Model file for the job. Use its own axes, mm. Face numbers are marked on the shaded views. A direction names the side the tool comes from. Round coordinates to 2 decimals unless told otherwise and drop trailing zeros. Loops run counter-clockwise (first coordinate to the right, second up) from the corner with the lowest first, then second, coordinate; pieces in that order, holes last. Notation, with made-up numbers: (7.25, -24.5) - (12.25, -24.5) arc R28 cw to (12.25, -4.5) - close; hole circle Ø7 at (-37, 58.25). An arc over 180 degrees is marked (long way). Answer as a JSON object with one key per item and string values.
from build123d import *

# Parameters (mm, degrees)
SKETCH1_R           = 12.7
SKETCH1_R_2         = 1.65
BOSS_EXTRUDE1_DEPTH = 12.7
SKETCH2_R           = 1.65
CUT_EXTRUDE1_DEPTH  = 12.7
SKETCH3_R           = 2.77495
CUT_EXTRUDE3_DEPTH  = 1.99898
SKETCH7_R           = 1.65
BOSS_EXTRUDE2_DEPTH = 10.70102
SKETCH8_R           = 1.65
BOSS_EXTRUDE3_DEPTH = 10.70102
SKETCH9_R           = 1.65
BOSS_EXTRUDE4_DEPTH = 10.70102
SKETCH10_R          = 1.65
BOSS_EXTRUDE5_DEPTH = 10.70102
SKETCH12_R          = 1.25
CUT_EXTRUDE4_DEPTH  = 12.7
SKETCH11_R          = 1.25
CUT_EXTRUDE5_DEPTH  = 12.7
SKETCH17_W          = 30.98386677
SKETCH17_H          = 12.7
BOSS_EXTRUDE6_DEPTH = 10.16
SKETCH18_R          = 1.650000002
SKETCH18_R_2        = 1.65
CUT_EXTRUDE6_DEPTH  = 24.384


with BuildPart() as part:
    # Sketch1 → Boss-Extrude1 (new body)
    with BuildSketch(Plane(origin=(0, 0, 0), x_dir=(1, 0, 0), z_dir=(0, 1, 0))):
        with BuildLine():
            Line((21.686311219, 59.206008809), (23.227161891, 57.665158137))
            ThreePointArc((23.227161891, 57.665158137), (23.323849078, 57.508955756), (23.357596674, 57.328376976))
            Line((23.357596674, 57.328376976), (23.357596674, 26.344510207))
            ThreePointArc((23.357596674, 26.344510207), (23.323849078, 26.163931427), (23.227161891, 26.007729046))
            Line((23.227161891, 26.007729046), (21.686311219, 24.466878374))
            ThreePointArc((21.686311219, 24.466878374), (21.530108838, 24.370191187), (21.349530059, 24.336443591))
            Line((21.349530059, 24.336443591), (-9.634336711, 24.336443591))
            ThreePointArc((-9.634336711, 24.336443591), (-9.814915491, 24.370191187), (-9.971117871, 24.466878374))
            Line((-9.971117871, 24.466878374), (-11.511968543, 26.007729046))
            ThreePointArc((-11.511968543, 26.007729046), (-11.60865573, 26.163931427), (-11.642403326, 26.344510207))
            Line((-11.642403326, 26.344510207), (-11.642403326, 57.328376976))
            ThreePointArc((-11.642403326, 57.328376976), (-11.60865573, 57.508955756), (-11.511968543, 57.665158137))
            Line((-11.511968543, 57.665158137), (-9.971117871, 59.206008809))
            ThreePointArc((-9.971117871, 59.206008809), (-9.814915491, 59.302695995), (-9.634336711, 59.336443591))
            Line((-9.634336711, 59.336443591), (21.349530059, 59.336443591))
            ThreePointArc((21.349530059, 59.336443591), (21.530108838, 59.302695995), (21.686311219, 59.206008809))
        make_face()
        with Locations(Location((5.857596674, 41.836443591, 0), (0, 0, 90))):
            Circle(SKETCH1_R, mode=Mode.SUBTRACT)
        with Locations(Location((18.857596674, 54.836443591, 0), (0, 0, 90))):
            Circle(SKETCH1_R_2, mode=Mode.SUBTRACT)
        with Locations(Location((18.857596674, 28.836443591, 0), (0, 0, 90))):
            Circle(SKETCH1_R_2, mode=Mode.SUBTRACT)
        with Locations(Location((-7.142403326, 54.836443591, 0), (0, 0, 90))):
            Circle(SKETCH1_R_2, mode=Mode.SUBTRACT)
        with Locations(Location((-7.142403326, 28.836443591, 0), (0, 0, 90))):
            Circle(SKETCH1_R_2, mode=Mode.SUBTRACT)
    extrude(amount=BOSS_EXTRUDE1_DEPTH)

    # Sketch2 → Cut-Extrude1 (cut)
    with BuildSketch(Plane.XY.offset(-24.336443591)):
        with Locations((-1.888370018, 6.35)):
            Circle(SKETCH2_R)
        with Locations((13.603563366, 6.35)):
            Circle(SKETCH2_R)
        with Locations((5.857596674, 6.35)):
            Circle(SKETCH2_R)
    extrude(amount=-CUT_EXTRUDE1_DEPTH, mode=Mode.SUBTRACT)

    # Sketch3 → Cut-Extrude3 (cut)
    with BuildSketch(Plane(origin=(0, 12.7, 0), x_dir=(1, 0, 0), z_dir=(0, 1, 0))):
        with Locations(Location((-7.142403326, 54.836443591, 0), (0, 0, 270))):
            Circle(SKETCH3_R)
        with Locations(Location((18.857596674, 54.836443591, 0), (0, 0, 270))):
            Circle(SKETCH3_R)
        with Locations(Location((-7.142403326, 28.836443591, 0), (0, 0, 270))):
            Circle(SKETCH3_R)
        with Locations(Location((18.857596674, 28.836443591, 0), (0, 0, 270))):
            Circle(SKETCH3_R)
    extrude(amount=-CUT_EXTRUDE3_DEPTH, mode=Mode.SUBTRACT)

    # Sketch7 → Boss-Extrude2 (add, through all)
    with BuildSketch(Plane(origin=(0, 10.70102, 0), x_dir=(1, 0, 0), z_dir=(0, 1, 0))):
        with Locations((-7.142403326, 28.836443591)):
            Circle(SKETCH7_R)
    extrude(amount=-BOSS_EXTRUDE2_DEPTH)

    # Sketch8 → Boss-Extrude3 (add, through all)
    with BuildSketch(Plane(origin=(0, 10.70102, 0), x_dir=(1, 0, 0), z_dir=(0, 1, 0))):
        with Locations((-7.142403326, 54.836443591)):
            Circle(SKETCH8_R)
    extrude(amount=-BOSS_EXTRUDE3_DEPTH)

    # Sketch9 → Boss-Extrude4 (add, through all)
    with BuildSketch(Plane(origin=(0, 10.70102, 0), x_dir=(1, 0, 0), z_dir=(0, 1, 0))):
        with Locations((18.857596674, 54.836443591)):
            Circle(SKETCH9_R)
    extrude(amount=-BOSS_EXTRUDE4_DEPTH)

    # Sketch10 → Boss-Extrude5 (add, through all)
    with BuildSketch(Plane(origin=(0, 10.70102, 0), x_dir=(1, 0, 0), z_dir=(0, 1, 0))):
        with Locations((18.857596674, 28.836443591)):
            Circle(SKETCH10_R)
    extrude(amount=-BOSS_EXTRUDE5_DEPTH)

    # Sketch12 → Cut-Extrude4 (cut)
    with BuildSketch(Plane(origin=(0, 10.70102, 0), x_dir=(1, 0, 0), z_dir=(0, 1, 0))):
        with Locations(Location((18.857596674, 54.836443591, 0), (0, 0, 270))):
            Circle(SKETCH12_R)
        with Locations(Location((-7.142403326, 28.836443591, 0), (0, 0, 270))):
            Circle(SKETCH12_R)
        with Locations(Location((18.857596674, 28.836443591, 0), (0, 0, 270))):
            Circle(SKETCH12_R)
    extrude(amount=-CUT_EXTRUDE4_DEPTH, mode=Mode.SUBTRACT)

    # Sketch11 → Cut-Extrude5 (cut)
    with BuildSketch(Plane(origin=(0, 10.70102, 0), x_dir=(1, 0, 0), z_dir=(0, 1, 0))):
        with Locations(Location((-7.142403326, 54.836443591, 0), (0, 0, 270))):
            Circle(SKETCH11_R)
    extrude(amount=-CUT_EXTRUDE5_DEPTH, mode=Mode.SUBTRACT)

    # Sketch17 → Boss-Extrude6 (add)
    with BuildSketch(Plane.XY.offset(-24.336443591)):
        with Locations((5.857596674, 6.35)):
            Rectangle(SKETCH17_W, SKETCH17_H)
    extrude(amount=BOSS_EXTRUDE6_DEPTH)

    # Sketch18 → Cut-Extrude6 (cut)
    with BuildSketch(Plane.XY.offset(-14.176443591)):
        with Locations((-1.888370018, 6.35)):
            Circle(SKETCH18_R)
        with Locations((5.857596674, 6.35)):
            Circle(SKETCH18_R_2)
        with Locations((13.603563366, 6.35)):
            Circle(SKETCH18_R_2)
    extrude(amount=-CUT_EXTRUDE6_DEPTH, mode=Mode.SUBTRACT)


solid = part.part
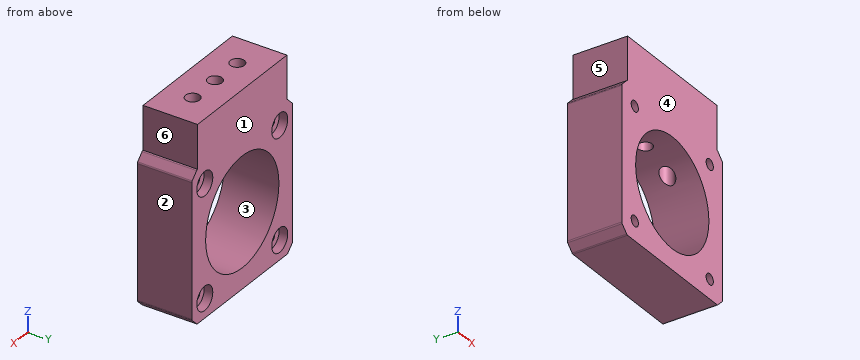
1) Tool access for the marked faces 4, 5 and 6: list every direction of +Z, -Z, +X, -X, +Y, -Y with a clear straight run to the whole face (end or side of a thin tool).
Values follow:
{"face 4": "+Z, -Z, +X, -X, -Y", "face 5": "+Z, -X, +Y, -Y", "face 6": "+Z, +X, +Y, -Y"}
2) Drop flat-ended pins along their axis: P1, Ø5, axis at y = 4.5, z = -20, coming from the -X side; P2, Ø3, axis at x = -7.14, z = -54.84, coming from the +Y side. Give the stop position or say it passes through.
Values follow:
{"P1": "x = -9.63", "P2": "y = 10.7"}
3) Slice it at A-A on x = 2.5. List the corners of the cut face in (y, z).
Values follow:
{"outline": "(0, -59.34) - (12.7, -59.34) - (12.7, -54.08) - (0, -54.08) - close; (0, -29.59) - (12.7, -29.59) - (12.7, -14.18) - (0, -14.18) - close"}
4) Slice it at C-C on z = -40.5. List the corners of the cut face in (x, y).
Values follow:
{"outline": "(-11.64, 0) - (-6.77, 0) - (-6.77, 12.7) - (-11.64, 12.7) - close; (18.49, 0) - (23.36, 0) - (23.36, 12.7) - (18.49, 12.7) - close"}
5) Two-plate mould, pull along X, no slides. Class the marked faces 1, 2 and 3: pulls with the +X half, pulls with the -X half, needs draft (parallel to the pull), parting line crosses it, or undercut.
Values follow:
{"face 1": "needs draft", "face 2": "pulls with the +X half", "face 3": "undercut"}
6) Probe probe 1 along X at (y, z) = (6.35, -18.75); probe 2 along Z at (x, y) = (19, 5.5); probe 3 along X at (y, z) = (11.75, -28.5). List the from-to ranges inside material, lowest first.
Values follow:
{"probe 1": "-9.63 to -3.54, -0.24 to 4.21, 7.51 to 11.95, 15.25 to 21.35", "probe 2": "-59.34 to -56.08, -53.59 to -30.08, -27.59 to -14.18", "probe 3": "-11.64 to -9.9, -4.39 to 16.1, 21.61 to 23.36"}
7) Slice it at B-B on y = 7.5. Count the separate pieces of the cut face and the enclosed holes in it, then the cut area to 3 significant figures.
Values follow:
{"separate pieces": "3", "enclosed holes": "4", "area": "888 mm²"}
8) Slice it at D-D on x = 13.5. List the corners of the cut face in (y, z), then the cut area to 3 significant figures.
Values follow:
{"outline": "(0, -59.34) - (12.7, -59.34) - (12.7, -51.98) - (0, -51.98) - close; (0, -31.69) - (4.7, -31.69) - (4.7, -14.18) - (0, -14.18) - close; (8, -31.69) - (12.7, -31.69) - (12.7, -14.18) - (8, -14.18) - close", "area": "258 mm²"}
